Source: CAD feature listing. Evaluate the final solid. Frame: model axes, mm. Face numbers are marked on the shaded views. Give positions to 0.01 mm unless a question says otherwise; leave off trailing zeros. Loops run counter-clockwise (first coordinate to the right, second up) from the corner with the lowest first, then second, coordinate; pieces in that order, holes last. Notation, with made-up numbers: (86.25, 74.5) -> (144.25, 74.5) arc R13 cw to (144.25, 81.5) -> close; hole circle Ø2 at (-11, 5.5). An arc over 180 degrees is marked (long way). Put each result on its own line as item: value.
```python
from build123d import *

# Parameters (mm, degrees)
SKETCH2_R           = 57.15
BOSS_EXTRUDE1_DEPTH = 6.35
SKETCH3_R           = 5.15
CUT_EXTRUDE1_DEPTH  = 7.35
CIRPATTERN1_COUNT   = 9
SKETCH6_R           = 1.7
CUT_EXTRUDE4_DEPTH  = 7.35
CIRPATTERN3_COUNT   = 6
SKETCH7_R           = 5.15
CUT_EXTRUDE5_DEPTH  = 7.35


with BuildPart() as part:
    # Sketch2 → Boss-Extrude1 (new body)
    with BuildSketch(Plane.XY):
        Circle(SKETCH2_R)
    extrude(amount=BOSS_EXTRUDE1_DEPTH)

    # Sketch3 → Cut-Extrude1 (cut, through all)
    with BuildSketch(Plane.XY.offset(6.35)):
        with Locations((0, 33)):
            Circle(SKETCH3_R)
    cut_extrude1 = extrude(amount=-CUT_EXTRUDE1_DEPTH, mode=Mode.SUBTRACT)

    # CirPattern1: Cut-Extrude1 ×9 about axis
    cirpattern1_axis = Axis((0, 0, 0), (0, 0, 1))
    for i in range(1, CIRPATTERN1_COUNT):
        add(cut_extrude1.rotate(cirpattern1_axis, i * 360 / CIRPATTERN1_COUNT), mode=Mode.SUBTRACT)

    # Sketch6 → Cut-Extrude4 (cut, through all)
    with BuildSketch(Plane.XY.offset(6.35)):
        with Locations((0, 53.975)):
            Circle(SKETCH6_R)
    cut_extrude4 = extrude(amount=-CUT_EXTRUDE4_DEPTH, mode=Mode.SUBTRACT)

    # CirPattern3: Cut-Extrude4 ×6 about axis
    cirpattern3_axis = Axis((0, 0, 0), (0, 0, 1))
    for i in range(1, CIRPATTERN3_COUNT):
        add(cut_extrude4.rotate(cirpattern3_axis, i * 360 / CIRPATTERN3_COUNT), mode=Mode.SUBTRACT)

    # Sketch7 → Cut-Extrude5 (cut, through all)
    with BuildSketch(Plane.XY.offset(6.35)):
        Circle(SKETCH7_R)
    extrude(amount=-CUT_EXTRUDE5_DEPTH, mode=Mode.SUBTRACT)


solid = part.part
```
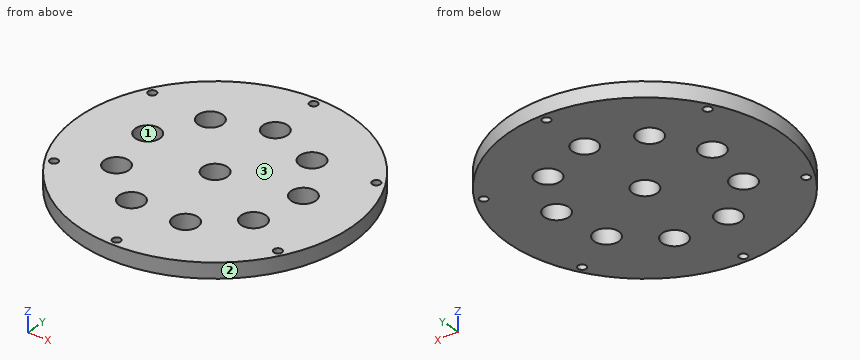
(1) Section D-D on y = -16.5. Return loops of the section in (x, z), then the cut area to 3 significant figures.
Calculated:
outline: (-54.72, 0) -> (-33.73, 0) -> (-33.73, 6.35) -> (-54.72, 6.35) -> close; (-23.43, 0) -> (23.43, 0) -> (23.43, 6.35) -> (-23.43, 6.35) -> close; (33.73, 0) -> (54.72, 0) -> (54.72, 6.35) -> (33.73, 6.35) -> close
area: 564 mm²
(2) Section B-B on y = 33. Return loops of the section in (x, z), then the cut area to 3 significant figures.
Calculated:
outline: (-46.66, 0) -> (-5.15, 0) -> (-5.15, 6.35) -> (-46.66, 6.35) -> close; (5.15, 0) -> (46.66, 0) -> (46.66, 6.35) -> (5.15, 6.35) -> close
area: 527 mm²
(3) Draft query along X for the marked faces 1, 2 and 3. Return one class per face: released by +X, released by -X, zero draft, split by the parting line, or undercut.
Calculated:
face 1: undercut
face 2: split by the parting line
face 3: zero draft
(4) First-contact query: P1, Ø3, axis at x = 25.5, y = 35, coming from the -Z side; P2, Ø3, axis at y = 5.5, z = 5, coming from the +X side; P3, Ø6, axis at x = 28.58, y = -16.5, coming from the -Z side; P4, Ø1, axis at x = 7, z = 1.5, coming from the -Y side. Flat tips, straight axial feed; report the tip coordinate or a pass-through.
Calculated:
P1: stops at z = 0
P2: stops at x = 57.01
P3: passes through
P4: stops at y = -56.78
(5) Section C-C on z = 2.5. Give the number of separate pieces and of enclosed holes in the cut face, then the cut area to 3 significant figures.
Calculated:
separate pieces: 1
enclosed holes: 16
area: 9,370 mm²
(6) Section A-A on x = -21.5. Return loops of the section in (y, z), then the cut area to 3 significant figures.
Calculated:
outline: (-52.95, 0) -> (20.14, 0) -> (20.14, 6.35) -> (-52.95, 6.35) -> close; (30.42, 0) -> (52.95, 0) -> (52.95, 6.35) -> (30.42, 6.35) -> close
area: 607 mm²
(7) Line query: probe 1 along Y at (x, z) = (0, 4.75) (3 decimals); probe 2 along X at (y, z) = (9, 6.25); probe 3 along X at (y, z) = (-0.5, 1.5). Output: solid intervals per line, ascending. Write a range as from..to.
Calculated:
probe 1: y = -57.15..-55.675, -52.275..-5.15, 5.15..27.85, 38.15..52.275, 55.675..57.15
probe 2: x = -56.44..-36.48, -28.52..28.52, 36.48..56.44
probe 3: x = -57.15..-5.13, 5.13..57.15
